```python
from build123d import *

# Parameters (mm, degrees)
F1_W      = 129
F1_H      = 92
F2_DEPTH  = 15
F4_W      = 129
F4_H      = 60
F5_DEPTH  = 11
F6_R      = 6
F3_W      = 8
F3_H      = 90
F3_W_2    = 7
F3_W_3    = 4
F3_W_4    = 12
F3_W_5    = 26
F7_DEPTH  = 14.6
F8_DEPTH  = 2
F9_DEPTH  = 2
F10_W     = 129
F10_H     = 60
F11_DEPTH = 25


with BuildPart() as f2:
    # F1 (on Top) → F2 (new body)
    with BuildSketch(Plane.XY):
        with Locations((6.5, 1)):
            Rectangle(F1_W, F1_H)
    extrude(amount=F2_DEPTH)

    # F4 (on face) → F5 (cut)
    with BuildSketch(Plane.XY.offset(15)):
        with Locations((6.5, 0)):
            Rectangle(F4_W, F4_H)
    extrude(amount=-F5_DEPTH, mode=Mode.SUBTRACT)

    # F6
    f6_edges = [f2.edges().sort_by_distance(p)[0] for p in [
        (6.5, 30, 15),
        (6.5, -30, 15),
    ]]
    fillet(f6_edges, radius=F6_R)

    # F3 (on face) → F7 (cut)
    with BuildSketch(Plane.XY.offset(15)):
        with Locations((-53, 1)):
            Rectangle(F3_W, F3_H)
        with Locations((-44.5, 1)):
            Rectangle(F3_W_2, F3_H)
        with Locations((-36.5, 1)):
            Rectangle(F3_W_2, F3_H)
        with Locations((-28.5, 1)):
            Rectangle(F3_W_2, F3_H)
        with Locations((-20.5, 1)):
            Rectangle(F3_W_2, F3_H)
        with Locations((-12.5, 1)):
            Rectangle(F3_W_2, F3_H)
        with Locations((-4.5, 1)):
            Rectangle(F3_W_2, F3_H)
        with Locations((3.5, 1)):
            Rectangle(F3_W_2, F3_H)
        with Locations((10, 1)):
            Rectangle(F3_W_3, F3_H)
        with Locations((15, 1)):
            Rectangle(F3_W_3, F3_H)
        with Locations((24, 1)):
            Rectangle(F3_W_4, F3_H)
        with Locations((37, 1)):
            Rectangle(F3_W_4, F3_H)
        with Locations((57, 1)):
            Rectangle(F3_W_5, F3_H)
    extrude(amount=-F7_DEPTH, mode=Mode.SUBTRACT)

    # F8 (add): a face of the model
    f8_faces = [f2.faces().sort_by_distance(p)[0] for p in [
        (-58, -40.5, 14.0678519431),
    ]]
    extrude(f8_faces, amount=F8_DEPTH)

    # F9 (add): a face of the model
    f9_faces = [f2.faces().sort_by_distance(p)[0] for p in [
        (71, 41.5, 14.0678519431),
    ]]
    extrude(f9_faces, amount=F9_DEPTH)

    # F10 (on face) → F11 (cut)
    with BuildSketch(Plane(origin=(0, 0, 0), x_dir=(1, 0, 0), z_dir=(0, 0, -1))):
        with Locations((6.5, 0)):
            Rectangle(F10_W, F10_H)
    extrude(amount=-F11_DEPTH, mode=Mode.SUBTRACT)


solid = f2.part
```
Input: part model. Units: mm. Frame: model coordinates. A direction names the side the tool comes from. Round coordinates to 2 decimals unless told otherwise and drop trailing zeros. Loops run counter-clockwise (first coordinate to the right, second up) from the corner with the lowest first, then second, coordinate; pieces in that order, holes last. Notation, with made-up numbers: (41.25, 57) -> (82.25, 57) arc R24 cw to (82.25, 96) -> close; hole circle Ø7 at (-27.75, -38). An arc over 180 degrees is marked (long way). Write each question's results on one line, items separated by ' | '.
1. Mould query, pull axis Z, two halves, no side actions, for faces 1 (the face through (-5, 38, 0.4)), 2 (the face through (-33, -37, 8)). Classes: +Z half, -Z half, draft (parallel to the pull), parting line (faces both ways), or undercut.
Geometry results:
face 1: +Z half | face 2: draft
2. Set-up query: faces 3 (the face through (6, 47, 7)), 4 (the face through (12.507, -31.711, 13.196)), 5 (the face through (-48, 38, 8)). Return all of +Z, -Z, +X, -X, +Y, -Y with unobstructed straight access to the full face (end or side cutting, diameter ignored); none if empty.
Geometry results:
face 3: +Z, -Z, +X, -X, +Y | face 4: +Z, +X, -X | face 5: +Z
3. First-contact query: P1, Ø10, axis at x = 45.5, y = 23, coming from the -Z side; P2, Ø8, axis at x = 7.5, y = -28, coming from the +Z side. Flat tips, straight axial feed; report the tip coordinate or a pass-through.
Geometry results:
P1: through | P2: z = 13.47
4. Section B-B (x = -12). Return loops of the section in (y, z), and give its area (3 significant figures).
Geometry results:
outline: (-45, 0) -> (-30, 0) -> (-30, 0.4) -> (-44, 0.4) -> (-44, 15) -> (-45, 15) -> close; (30, 0) -> (47, 0) -> (47, 15) -> (46, 15) -> (46, 0.4) -> (30, 0.4) -> close | area: 42.0 mm2
5. Section A-A (y = 9). Return loops of the section in (x, z).
Geometry results:
outline: (-60, 0) -> (-58, 0) -> (-58, 4) -> (-60, 4) -> close; (71, 0) -> (73, 0) -> (73, 4) -> (71, 4) -> close
6. Ray query, line 1 (X direction, y = 28, z = 2.5); line 2 (Y direction, x = -21, z = 12); line 3 (Z direction, x = -19, y = 42.5). Return the intervals inside material, ascending. Write a range as from..to.
Geometry results:
line 1: -60..-58, 71..73 | line 2: -45..-44, 46..47 | line 3: 0..0.4
